For this review, take the finished solid that the model builds, in its own axes (mm). Coordinates: 2 decimals unless noted, no trailing zeros. Loops run counter-clockwise (first coordinate to the right, second up) from the corner with the lowest first, then second, coordinate; pieces in that order, holes last. Notation, with made-up numbers: (54, -26) -> (60, -26) arc R30 cw to (60, 5) -> close; hole circle Ø7 at (-36.5, 72). An arc over 180 degrees is marked (long way). One line per item, written item: value.
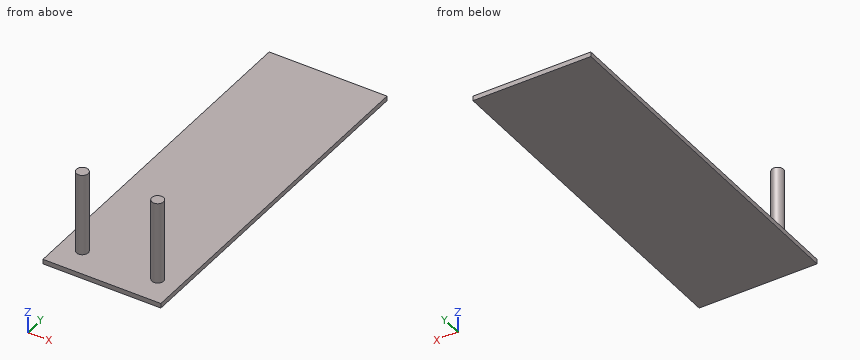
from build123d import *

# Parameters (mm, degrees)
F0_W     = 50
F0_H     = 150
F1_DEPTH = 2
F2_R     = 2.5
F3_DEPTH = 35


# Not quite as in the source:
# - a pattern or mirror of a feature is missing from the dataset's text; its kind, count and spacing are read off the source's solid


with BuildPart() as f1:
    # F0 (on Top) → F1 (new body)
    with BuildSketch(Plane.XY):
        Rectangle(F0_W, F0_H)
    extrude(amount=F1_DEPTH)

    # F2 (on face) → F3 (join)
    with BuildSketch(Plane.XY.offset(2)):
        with Locations((-16, -63)):
            Circle(F2_R)
    f3 = extrude(amount=F3_DEPTH)

    # F3_copies: F3 across plane
    add(f3.mirror(Plane(origin=(0, 0, 0), x_dir=(0, 0, 1), z_dir=(1, 0, 0))))


solid = f1.part
1. Take a section at A-A, the plane y = -63. Give the boundary of the cut face in (x, z).
Return value:
outline: (-25, 0) -> (25, 0) -> (25, 2) -> (18.5, 2) -> (18.5, 37) -> (13.5, 37) -> (13.5, 2) -> (-13.5, 2) -> (-13.5, 37) -> (-18.5, 37) -> (-18.5, 2) -> (-25, 2) -> close
2. To check wall thickness, follow probe 1 along Z at (x, y) = (-3, 16.5); probe 2 along Y at (x, z) = (-15, 32); probe 3 along Y at (x, z) = (-16.5, 3). State the ranges of each line that lie inside material, in increasing order. Write a range as from..to.
Return value:
probe 1: z = 0..2
probe 2: y = -65.29..-60.71
probe 3: y = -65.45..-60.55
3. Insertion check: pin 1 Ø6 at (x, z) = (-18.5, 32.5) entering from +Y; pin 2 Ø1 at (x, z) = (-17, 33) entering from -Y; pin 3 Ø15 at (x, y) = (-6, -28) entering from +Z. Each pin has a flat end and moves straight along its axis. Give the tip position at first contact, or say it passes through.
Return value:
pin 1: stops at y = -60.5
pin 2: stops at y = -65.45
pin 3: stops at z = 2
4. Take a section at C-C, the plane x = 16. Give the boundary of the cut face in (y, z), and give its area (3 significant figures).
Return value:
outline: (-75, 0) -> (75, 0) -> (75, 2) -> (-60.5, 2) -> (-60.5, 37) -> (-65.5, 37) -> (-65.5, 2) -> (-75, 2) -> close
area: 475 mm2
5. Take a section at B-B, the plane z = 21. Give the boundary of the cut face in (x, y), and give its area (3 significant figures).
Return value:
outline: circle Ø5 at (-16, -63); circle Ø5 at (16, -63)
area: 39.3 mm2
6. Take a section at D-D, the plane y = 23. Give the boundary of the cut face in (x, z), and give its area (3 significant figures).
Return value:
outline: (-25, 0) -> (25, 0) -> (25, 2) -> (-25, 2) -> close
area: 100 mm2
